The drawing under review shows one solid part. Ordinate dimensions are in mm from its lowest x, y, z. Give positions to 0.01 mm unless a question says otherwise; leave off trailing zeros. Order: outer loops, then holes, each group sorted by start corner. A loop starts at its lowest first (then second) coordinate and runs counter-clockwise, first axis right, second up. Notation, with made-up numbers: (44.5, 16) -> (59.5, 16) arc R12 ccw to (59.5, 24) -> close; hole circle Ø1 at (-11.75, 44). An arc over 180 degrees is marked (long way). One line per item, written item: value. Start each with the question number.
1) Consider section A-A (x = 44.5). State the section outline as (y, z) points, plus the area to 3 significant figures.
2) The part is to be moulded in two halves that separate along Y. For the marked faces 1, 2 and 3, say which applies: released by +Y, released by -Y, zero draft, split by the parting line, or undercut.
3) Consider section D-D (z = 4). State the section outline as (x, y) points.
4) For pin 1 (4 mm diameter, centred on y = 44.5, z = 4, fed in from +X); pin 2 (1.5 mm diameter, centred on y = 65, z = 3.5, fed in from -X); pin 3 (0.9 mm diameter, centred on y = 44.5, z = 3.5, fed in from +X); pin 4 (0.9 mm diameter, centred on y = 45, z = 4.5, fed in from -X), all flat-tipped, find the tip position at first contact; note any pin that passes through.
5) Consider section C-C (y = 60.5). State the section outline as (x, z) points.
6) Wall thickness on line 1 along Y through (x, z) = (44.5, 3.5); line 2 along Y through (x, z) = (44.5, 2.25); line 3 along Y through (x, z) = (51.5, 4.5): over which ranges is each line inside the solid? List them lowest first. Write a range as from..to.
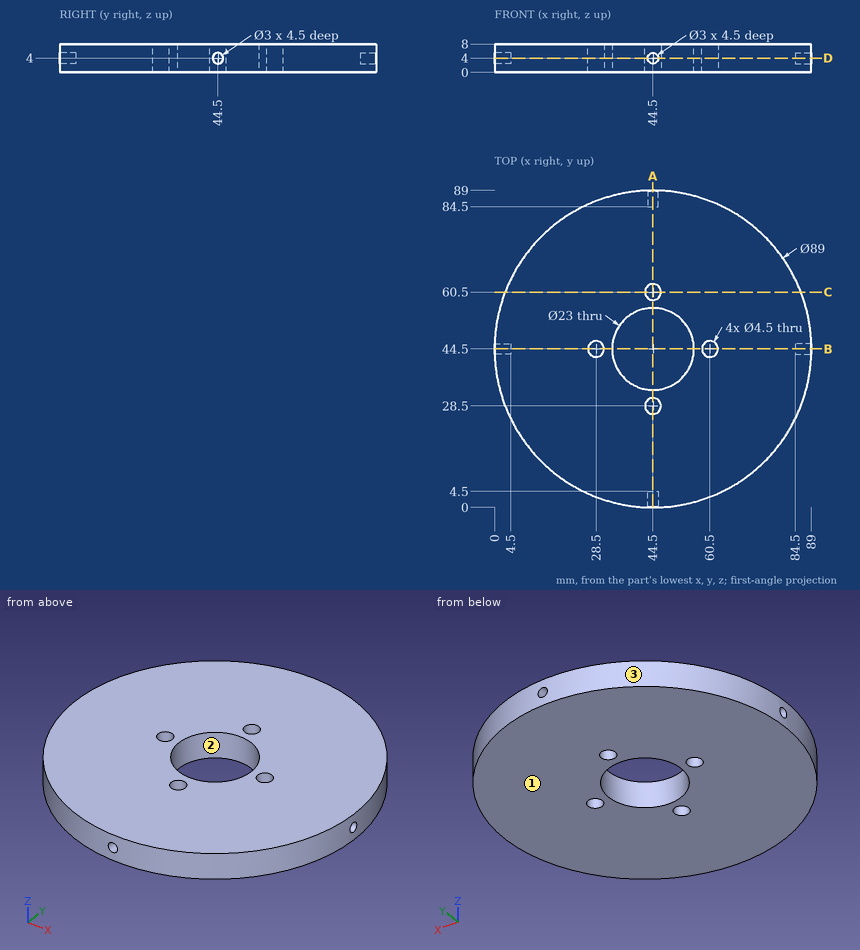
Checked values:
1. outline: (0, 0) -> (26.25, 0) -> (26.25, 8) -> (0, 8) -> (0, 5.5) -> (4.5, 5.5) -> (4.5, 2.5) -> (0, 2.5) -> close; (30.75, 0) -> (33, 0) -> (33, 8) -> (30.75, 8) -> close; (56, 0) -> (58.25, 0) -> (58.25, 8) -> (56, 8) -> close; (62.75, 0) -> (89, 0) -> (89, 2.5) -> (84.5, 2.5) -> (84.5, 5.5) -> (89, 5.5) -> (89, 8) -> (62.75, 8) -> close
1. area: 429 mm^2
2. face 1: zero draft
2. face 2: undercut
2. face 3: split by the parting line
3. outline: (0.03, 43) arc R44.5 ccw to (43, 0.03) -> (43, 4.5) -> (46, 4.5) -> (46, 0.03) arc R44.5 ccw to (88.97, 43) -> (84.5, 43) -> (84.5, 46) -> (88.97, 46) arc R44.5 ccw to (46, 88.97) -> (46, 84.5) -> (43, 84.5) -> (43, 88.97) arc R44.5 ccw to (0.03, 46) -> (4.5, 46) -> (4.5, 43) -> close; hole circle Ø4.5 at (28.5, 44.5); hole circle Ø23 at (44.5, 44.5); hole circle Ø4.5 at (44.5, 28.5); hole circle Ø4.5 at (44.5, 60.5); hole circle Ø4.5 at (60.5, 44.5)
4. pin 1: stops at x = 89
4. pin 2: stops at x = 4.62
4. pin 3: stops at x = 84.5
4. pin 4: stops at x = 4.5
5. outline: (2.98, 0) -> (42.25, 0) -> (42.25, 8) -> (2.98, 8) -> close; (46.75, 0) -> (86.02, 0) -> (86.02, 8) -> (46.75, 8) -> close
6. line 1: y = 4.5..26.25, 30.75..33, 56..58.25, 62.75..84.5
6. line 2: y = 0..26.25, 30.75..33, 56..58.25, 62.75..89
6. line 3: y = 0.55..35.38, 53.62..88.45
